For this review, take the finished solid that the model builds, in its own axes (mm). Face numbers are marked on the shaded views. A direction names the side the tool comes from. Give positions to 0.01 mm unless a question says otherwise; leave off trailing zeros. Answer as CSV lines item,"result".
from build123d import *

# Parameters (mm, degrees)
SKETCH1_R           = 19.05
BOSS_EXTRUDE1_DEPTH = 104.775
CUT_EXTRUDE1_DEPTH  = 104.775


with BuildPart() as part:
    # Sketch1 → Boss-Extrude1 (new body)
    with BuildSketch(Plane(origin=(0, 0, 0), x_dir=(1, 0, 0), z_dir=(0, 1, 0))):
        Circle(SKETCH1_R)
    extrude(amount=BOSS_EXTRUDE1_DEPTH)

    # Sketch2 → Cut-Extrude1 (cut)
    with BuildSketch(Plane.XZ):
        Polygon((-15.323636661, -1.510781079), (-6.353443536, -14.026049167), (8.970193125, -12.515268087), (15.323636661, 1.510781079), (6.353443536, 14.026049167), (-8.970193125, 12.515268087), align=None)
    extrude(amount=-CUT_EXTRUDE1_DEPTH, mode=Mode.SUBTRACT)

    # Sketch4 → Revolve1 (revolve)
    with BuildSketch(Plane.XY):
        with BuildLine():
            Line((-19.05, 104.775), (-19.05, 0))
            ThreePointArc((-19.05, 0), (-31.75, 52.3875), (-19.05, 104.775))
        make_face()
    revolve(axis=Axis((0, 0, 0), (0, 1, 0)))


solid = part.part
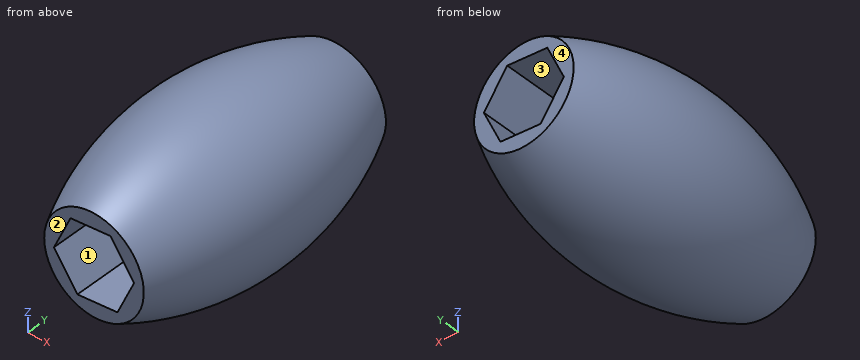
1) Machinability: for the marked faces 3 and 4, which of the approach directions +Z, -Z, +X, -X, +Y, -Y give a long, thin tool a straight path to every point of the face, cutting with its end or side? Answer none if there is none.
From the geometry:
face 3,"+Y, -Y"
face 4,"+Z, -Z, +X, -X, +Y"
2) Wall thickness on line 1 (Z direction, x = 2.5, y = 26.5); line 2 (Z direction, x = -15, y = 75); line 3 (X direction, y = 42.5, z = -4.5): over which ranges is each line inside the solid? List them lowest first. Write a range as from..to.
From the geometry:
line 1,"z = -28.67..-13.15, 13.65..28.67"
line 2,"z = -25.39..-1.96, -0.8..25.39"
line 3,"x = -31..-13.18, 12.6..31"
3) Draft analysis for pull direction X (two halves, no side actions). For the marked faces 1 and 2, state which applies: pulls with the +X half, pulls with the -X half, needs draft (parallel to the pull), parting line crosses it, or undercut.
From the geometry:
face 1,"undercut"
face 2,"needs draft"
4) Insertion check: P1, Ø6, axis at x = -12.5, z = 15.5, coming from the -Y side; P2, Ø3, axis at x = -1.5, y = 83.5, coming from the +Z side; P3, Ø12, axis at x = 5, y = 47.5, coming from the +Z side; P4, Ø8, axis at x = -6, y = 13, coming from the -Z side. Each pin has a flat end and moves straight along its axis. Give the tip position at first contact, or say it passes through.
From the geometry:
P1,"stops at y = 0"
P2,"stops at z = 27.82"
P3,"stops at z = 31.74"
P4,"stops at z = -25.66"
